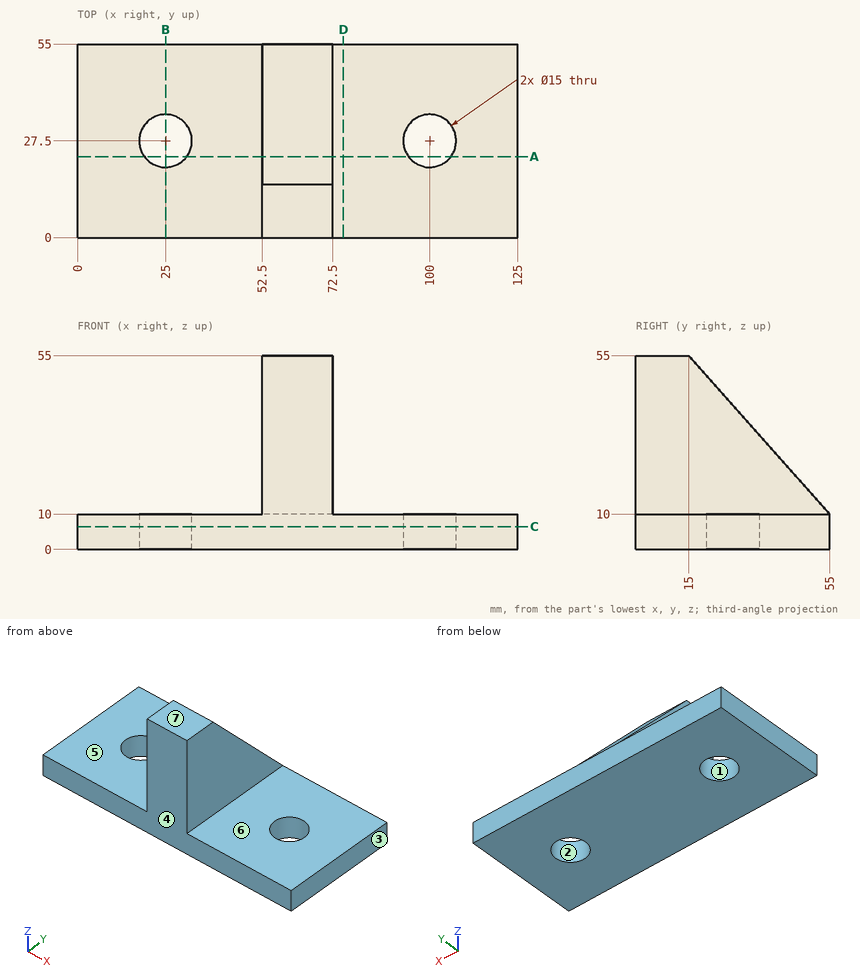
Design review of the part shown in the three views and the two pictorial views. Dimensions are in mm from the part's minimum x, y and z. A direction names the side the tool comes from. Coordinates: 2 decimals unless noted, no trailing zeros. Loops run counter-clockwise (first coordinate to the right, second up) from the corner with the lowest first, then second, coordinate; pieces in that order, holes last.
(1) Insertion check: P1, Ø1.5, axis at y = 40, z = 25, coming from the -X side; P2, Ø1, axis at x = 64.5, z = 28, coming from the -Y side; P3, Ø8, axis at x = 75.5, z = 30.5, coming from the +Y side; P4, Ø1.5, axis at x = 62.5, z = 29, coming from the +Y side. Each pin has a flat end and moves straight along its axis. Give the tip position at first contact, or say it passes through.
Determined:
P1: stops at x = 52.5
P2: stops at y = 0
P3: stops at y = 39.13
P4: stops at y = 38.78
(2) Consider section A-A, the plane y = 23. Give the boundary of the cut face in (x, z), plus the area to 3 significant figures.
Determined:
outline: (0, 0) - (19, 0) - (19, 10) - (0, 10) - close; (31, 0) - (94, 0) - (94, 10) - (72.5, 10) - (72.5, 46) - (52.5, 46) - (52.5, 10) - (31, 10) - close; (106, 0) - (125, 0) - (125, 10) - (106, 10) - close
area: 1,730 mm2
(3) Consider section B-B, the plane x = 25. Give the boundary of the cut face in (y, z).
Determined:
outline: (0, 0) - (20, 0) - (20, 10) - (0, 10) - close; (35, 0) - (55, 0) - (55, 10) - (35, 10) - close
(4) Tool access review of the marked faces 5, 6 and 7: name each direction out of +Z, -Z, +X, -X, +Y, -Y from which nothing blocks a thin tool from reaching the whole face with its end or side.
Determined:
face 5: +Z, -X, +Y, -Y
face 6: +Z, +X, +Y, -Y
face 7: +Z, +X, -X, +Y, -Y
(5) Consider section D-D, the plane x = 75.5. Give the boundary of the cut face in (y, z).
Determined:
outline: (0, 0) - (55, 0) - (55, 10) - (0, 10) - close
(6) Draft analysis for pull direction Y (two halves, no side actions). For the marked faces 1, 2, 3 and 4, state which applies: +Y half, -Y half, draft (parallel to the pull), parting line (faces both ways), or undercut.
Determined:
face 1: undercut
face 2: undercut
face 3: draft
face 4: -Y half
(7) Wall thickness on L1, parallel to X at y = 27, z = 5; L2, parallel to Y at x = 25, z = 6; L3, parallel to Z at x = 92.5, y = 6: over which ranges is each line inside the solid? List them lowest first.
Determined:
L1: x = 0 to 17.52, 32.48 to 92.52, 107.48 to 125
L2: y = 0 to 20, 35 to 55
L3: z = 0 to 10
(8) Consider section C-C, the plane z = 6.5. Give the boundary of the cut face in (x, y), plus the area to 3 significant figures.
Determined:
outline: (0, 0) - (125, 0) - (125, 55) - (0, 55) - close; hole circle Ø15 at (25, 27.5); hole circle Ø15 at (100, 27.5)
area: 6,520 mm2
